Here's how the part is built. I have some questions about the finished solid (model axes, mm). A direction names the side the tool comes from. Coordinates: 2 decimals unless noted, no trailing zeros. Write each loop counter-clockwise with the first axis right and the second up, starting at its lowest first coordinate (ties: lowest second). Pieces come first, ordered by that corner, then holes. Notation, with made-up numbers: M 82.25,79 L 120.25,79 A31 cw 120.25,113 Z; hole C 42,88 d10. An arc over 180 degrees is marked long. Write each question's results on one line, items separated by ' | '. Start each with the question number.
from build123d import *

# Parameters (mm, degrees)
SKETCH1_R           = 7.99
BOSS_EXTRUDE1_DEPTH = 1
FILLET1_R           = 0.2
SKETCH2_R           = 2.99
BOSS_EXTRUDE3_DEPTH = 58
SKETCH4_R           = 1.5
BOSS_EXTRUDE4_DEPTH = 2
SKETCH5_R           = 2.99
BOSS_EXTRUDE5_DEPTH = 1


with BuildPart() as part:
    # Sketch1 → Boss-Extrude1 (new body)
    with BuildSketch(Plane(origin=(0, 0, 0), x_dir=(1, 0, 0), z_dir=(0, 1, 0))):
        with Locations(Location((0, 0, 0), (0, 0, 270))):
            Circle(SKETCH1_R)
    extrude(amount=BOSS_EXTRUDE1_DEPTH)

    # Fillet1
    fillet1_edges = [part.edges().sort_by_distance(p)[0] for p in [
        (0, 0, -7.99),
        (0, 1, -7.99),
    ]]
    fillet(fillet1_edges, radius=FILLET1_R)

    # Sketch2 → Boss-Extrude3 (add)
    with BuildSketch(Plane(origin=(0, 1, 0), x_dir=(1, 0, 0), z_dir=(0, 1, 0))):
        with Locations(Location((0, 0, 0), (0, 0, 90))):
            Circle(SKETCH2_R)
    extrude(amount=BOSS_EXTRUDE3_DEPTH)

    # Sketch4 → Boss-Extrude4 (add)
    with BuildSketch(Plane(origin=(0, 59, 0), x_dir=(1, 0, 0), z_dir=(0, 1, 0))):
        with Locations(Location((0, 0, 0), (0, 0, 270))):
            Circle(SKETCH4_R)
    extrude(amount=BOSS_EXTRUDE4_DEPTH)

    # Sketch5 → Boss-Extrude5 (add)
    with BuildSketch(Plane(origin=(0, 61, 0), x_dir=(1, 0, 0), z_dir=(0, 1, 0))):
        with Locations(Location((0, 0, 0), (0, 0, 90))):
            Circle(SKETCH5_R)
    extrude(amount=BOSS_EXTRUDE5_DEPTH)


solid = part.part
1) We'd pull the mould along Y, two halves only. Please class faces 4 (the flat face through (0, 62, 0)), 5 (the cylindrical face through (0.45, 59.99, 1.43)), 6 (the flat face through (0, 0, 0)), 7 (the flat face through (1.3, 59, -1.3)): pulls with the +Y half, pulls with the -Y half, needs draft (parallel to the pull), parting line crosses it, or undercut.
2) For faces 1 (the flat face through (1.3, 61, -1.3)), 2 (the cylindrical face through (-7.8, 0.5, -1.73)), 3 (the flat face through (0.1, 1, 3.4)), which set-ups out of +Z, -Z, +X, -X, +Y, -Y let a thin tool reach every point of the face, with its end or its side?
3) I want a section at C-C, the plane y = 34. Write out the boundary of the cut face in (x, z), then the cut area to 3 significant figures.
4) I want a section at A-A, the plane z = 0. Write out the boundary of the cut face in (x, y).
5) For pin 1 Ø1.5 at (x, z) = (5.5, 3.5) entering from -Y; pin 2 Ø1.5 at (x, y) = (-5.5, 24.5) entering from +Z; pin 3 Ø8 at (x, y) = (3.5, 39.5) entering from -Z; pin 4 Ø3 at (x, y) = (-1, 53.5) entering from +Z, each with a flat end and sliding along its axis, tell me the tip position at first contact or that it passes through.
6) Please list where these lines run through material, in increasing order: line 1 (Y direction, x = -4.75, z = 5); line 2 (Z direction, x = 1.5, y = 16); line 3 (X direction, y = 58, z = -2.75). Write a range as [from, to].
7) I want a section at B-B, the plane x = 0. Write out the boundary of the cut face in (y, z).
Output:
1) face 4: pulls with the +Y half | face 5: undercut | face 6: pulls with the -Y half | face 7: undercut
2) face 1: none | face 2: +Y, -Y | face 3: +Y
3) outline: C 0,0 d5.98 | area: 28.1 mm2
4) outline: M -7.99,0.2 A0.2 ccw -7.79,0 L 7.79,0 A0.2 ccw 7.99,0.2 L 7.99,0.8 A0.2 ccw 7.79,1 L 2.99,1 L 2.99,59 L 1.5,59 L 1.5,61 L 2.99,61 L 2.99,62 L -2.99,62 L -2.99,61 L -1.5,61 L -1.5,59 L -2.99,59 L -2.99,1 L -7.79,1 A0.2 ccw -7.99,0.8 Z
5) pin 1: stops at y = 0 | pin 2: passes through | pin 3: stops at z = -2.99 | pin 4: stops at z = 2.99
6) line 1: y = [0, 1] | line 2: z = [-2.59, 2.59] | line 3: x = [-1.17, 1.17]
7) outline: M 0,-7.79 A0.2 ccw 0.2,-7.99 L 0.8,-7.99 A0.2 ccw 1,-7.79 L 1,-2.99 L 59,-2.99 L 59,-1.5 L 61,-1.5 L 61,-2.99 L 62,-2.99 L 62,2.99 L 61,2.99 L 61,1.5 L 59,1.5 L 59,2.99 L 1,2.99 L 1,7.79 A0.2 ccw 0.8,7.99 L 0.2,7.99 A0.2 ccw 0,7.79 Z
